Here's how the part is built. I have some questions about the finished solid (model axes, mm). Face numbers are marked on the shaded views. A direction names the side the tool comes from. Coordinates: 2 decimals unless noted, no trailing zeros. Write each loop counter-clockwise with the first axis right and the second up, starting at its lowest first coordinate (ties: lowest second). Pieces come first, ordered by that corner, then holes.
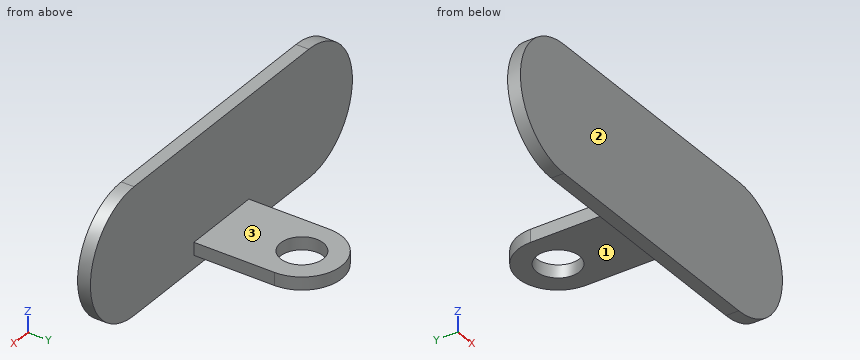
from build123d import *

# Parameters (mm, degrees)
SKETCH1_W           = 55.88
SKETCH1_H           = 9
BOSS_EXTRUDE1_DEPTH = 9
SKETCH2_R           = 15
BOSS_EXTRUDE2_DEPTH = 9


with BuildPart() as part:
    # Sketch1 → Boss-Extrude1 (new body)
    with BuildSketch(Plane(origin=(0, 0, 0), x_dir=(1, 0, 0), z_dir=(0, 1, 0))):
        with BuildLine():
            Line((-88.9, -44.323), (88.9, -44.323))
            ThreePointArc((88.9, -44.323), (133.223, 0), (88.9, 44.323))
            Line((88.9, 44.323), (-88.9, 44.323))
            ThreePointArc((-88.9, 44.323), (-133.223, 0), (-88.9, -44.323))
        make_face()
        with Locations((0, 30.823)):
            Rectangle(SKETCH1_W, SKETCH1_H, mode=Mode.SUBTRACT)
    extrude(amount=BOSS_EXTRUDE1_DEPTH)

    # Sketch2 → Boss-Extrude2 (add)
    with BuildSketch(Plane.XY.offset(-35.323)):
        with BuildLine():
            Line((-27.94, 0), (27.94, 0))
            Line((27.94, 0), (27.94, 65.532))
            ThreePointArc((27.94, 65.532), (0, 93.472), (-27.94, 65.532))
            Line((-27.94, 65.532), (-27.94, 0))
        make_face()
        with Locations((0, 65.532)):
            Circle(SKETCH2_R, mode=Mode.SUBTRACT)
    extrude(amount=BOSS_EXTRUDE2_DEPTH)


solid = part.part
1. I want a section at B-B (y = 75). List the corners of the cut face in (x, z) for me, then the cut area to 3 significant figures.
2. If I drill on line 1 (Y direction, x = 0, z = -31); line 2 (Y direction, x = 64, z = -2); line 3 (Z direction, x = 99, y = 5), over which ranges is the centre line in solid material (lowest first)?
3. I want a section at C-C (z = -30). List the corners of the cut face in (x, y) for me, then the cut area to 3 significant figures.
4. On a 3-axis mill with a long thin cutter (end or side, diameter ignored), from which of +Z, -Z, +X, -X, +Y, -Y can I reach the whole of each face in a straight line? I mean the marked faces 1, 2 and 3. Say none if no direction works.
5. For pin 1 Ø1.5 at (x, z) = (64, 27.5) entering from +Y; pin 2 Ø7 at (y, z) = (42.5, -32.5) entering from -X; pin 3 Ø7 at (y, z) = (38, -31.5) entering from +X, each with a flat end and sliding along its axis, tell me the tip position at first contact or that it passes through.
6. I want a section at D-D (x = -38). List the corners of the cut face in (y, z) for me.
7. I want a section at A-A (x = 0). List the corners of the cut face in (y, z) for me.
Response values:
1. outline: (-26.29, -35.32) - (-11.63, -35.32) - (-11.63, -26.32) - (-26.29, -26.32) - close; (11.63, -35.32) - (26.29, -35.32) - (26.29, -26.32) - (11.63, -26.32) - close
1. area: 264 mm2
2. line 1: y = 0 to 50.53, 80.53 to 93.47
2. line 2: y = 0 to 9
2. line 3: z = -43.16 to 43.16
3. outline: (-121.53, 0) - (121.53, 0) - (121.53, 9) - (27.94, 9) - (27.94, 65.53) arc R27.94 ccw to (-27.94, 65.53) - (-27.94, 9) - (-121.53, 9) - close; hole circle Ø30 at (0, 65.53)
3. area: 5,870 mm2
4. face 1: -Z, +X, -X, +Y
4. face 2: +Z, -Z, +X, -X, -Y
4. face 3: +Z, +X, -X, +Y
5. pin 1: stops at y = 9
5. pin 2: stops at x = -27.94
5. pin 3: stops at x = 27.94
6. outline: (0, -44.32) - (9, -44.32) - (9, 44.32) - (0, 44.32) - close
7. outline: (0, -44.32) - (9, -44.32) - (9, -35.32) - (50.53, -35.32) - (50.53, -26.32) - (9, -26.32) - (9, 44.32) - (0, 44.32) - close; (80.53, -35.32) - (93.47, -35.32) - (93.47, -26.32) - (80.53, -26.32) - close
